Design review of the part built by this model. Coordinates are the model's own, in mm. A direction names the side the tool comes from. Give positions to 0.01 mm unless a question says otherwise; leave off trailing zeros. Write each loop counter-clockwise with the first axis right and the second up, starting at its lowest first coordinate (ties: lowest second). Pieces come first, ordered by that corner, then holes. Notation, with made-up numbers: (13.25, -24.5) -> (19.25, -24.5) arc R23 ccw to (19.25, -13.5) -> close; hole circle Ø3 at (68, 68). An arc over 180 degrees is marked (long way). Return JSON: item names as keys, results as strings. Group by question number.
from build123d import *

# Parameters (mm, degrees)
F0_W     = 25.4
F0_H     = 25.4
F1_DEPTH = 155.8544
F2_W     = 22.2504
F2_H     = 22.2504
F3_DEPTH = 155.8544
F4_R     = 1.524
F5_R     = 0.254


with BuildPart() as f1:
    # F0 (on Front) → F1 (new body)
    with BuildSketch(Plane.XZ):
        Rectangle(F0_W, F0_H)
    extrude(amount=F1_DEPTH)

    # F2 (on face) → F3 (cut, through all)
    with BuildSketch(Plane.XZ.offset(155.8544)):
        Rectangle(F2_W, F2_H)
    extrude(amount=-F3_DEPTH, mode=Mode.SUBTRACT)

    # F4
    f4_edges = [f1.edges().sort_by_distance(p)[0] for p in [
        (-11.1252, -77.9272, 11.1252),
        (11.1252, -77.9272, -11.1252),
        (11.1252, -77.9272, 11.1252),
        (-11.1252, -77.9272, -11.1252),
    ]]
    fillet(f4_edges, radius=F4_R)

    # F5
    f5_edges = [f1.edges().sort_by_distance(p)[0] for p in [
        (12.7, -77.9272, 12.7),
        (12.7, -77.9272, -12.7),
        (-12.7, -77.9272, -12.7),
        (-12.7, -77.9272, 12.7),
    ]]
    fillet(f5_edges, radius=F5_R)


solid = f1.part
Q1. Mouldability with a two-part tool opening along Z and no side actions: class faces 3 (the face through (-11.3, -155.854, 0.1)), 4 (the face through (0, -77, -12.7)), 5 (the face through (0, -79, -11.125)) as +Z half, -Z half, draft (parallel to the pull), parting line (faces both ways), or undercut.
Q2. Take a section at C-C, the plane y = -132.5. Give the boundary of the cut face in (x, z), plus the area to 3 significant figures.
Q3. Tool access review of faces 1 (the face through (0, -79, 11.125)), 2 (the face through (12.7, -77, 0)): name each direction out of +Z, -Z, +X, -X, +Y, -Y from which nothing blocks a thin tool from reaching the whole face with its end or side.
Q4. Take a section at A-A, the plane z = 5.5. Give the boundary of the cut face in (x, y), plus the area to 3 significant figures.
Q5. For L1, parallel to Z at x = -5.25, y = -72; L2, parallel to Z at x = -10.25, y = -139.5, list the stretches that pass through material, from the lowest coordinate up. Write a range as from..to.
Q6. Insertion check: pin 1 (1.5 mm diameter, centred on x = -5.5, z = 9.5, fed in from +Y). The pin has a flat end and moves straight along its axis. Give the tip position at first contact, or say it passes through.
Q7. Take a section at B-B, the plane x = -1. Give the boundary of the cut face in (y, z), plus the area to 3 significant figures.
Final values:
{
 "1": {"face 3": "draft", "face 4": "-Z half", "face 5": "undercut"},
 "2": {"outline": "(-12.7, -12.45) arc R0.25 ccw to (-12.45, -12.7) -> (12.45, -12.7) arc R0.25 ccw to (12.7, -12.45) -> (12.7, 12.45) arc R0.25 ccw to (12.45, 12.7) -> (-12.45, 12.7) arc R0.25 ccw to (-12.7, 12.45) -> close; hole (-11.13, -9.6) arc R1.52 ccw to (-9.6, -11.13) -> (9.6, -11.13) arc R1.52 ccw to (11.13, -9.6) -> (11.13, 9.6) arc R1.52 ccw to (9.6, 11.13) -> (-9.6, 11.13) arc R1.52 ccw to (-11.13, 9.6) -> close", "area": "152 mm²"},
 "3": {"face 1": "+Y, -Y", "face 2": "+Z, -Z, +X, +Y, -Y"},
 "4": {"outline": "(-12.7, -155.85) -> (-11.13, -155.85) -> (-11.13, 0) -> (-12.7, 0) -> close; (11.13, -155.85) -> (12.7, -155.85) -> (12.7, 0) -> (11.13, 0) -> close", "area": "491 mm²"},
 "5": {"L1": "z = -12.7..-11.13, 11.13..12.7", "L2": "z = -12.7..-10.98, 10.98..12.7"},
 "6": {"pin 1": "passes through"},
 "7": {"outline": "(-155.85, -12.7) -> (0, -12.7) -> (0, -11.13) -> (-155.85, -11.13) -> close; (-155.85, 11.13) -> (0, 11.13) -> (0, 12.7) -> (-155.85, 12.7) -> close", "area": "491 mm²"}
}
